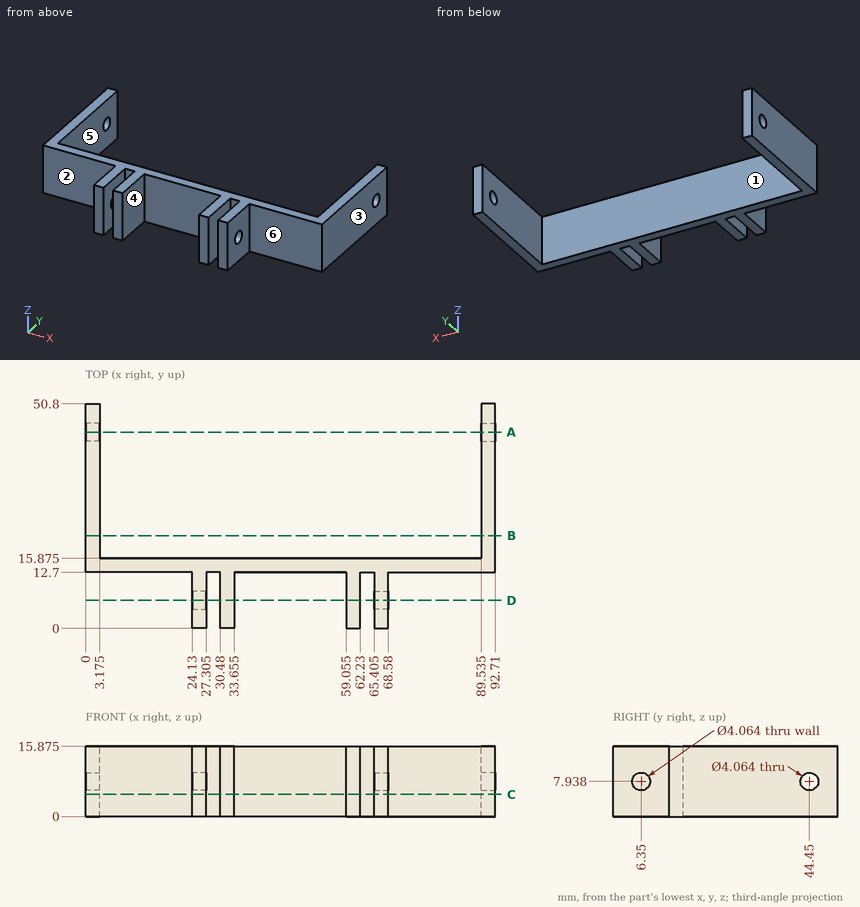
Part print with two shaded views. Sizes in mm from the minimum x, y, z corner. A direction names the side the tool comes from. Give positions to 0.01 mm unless a question says otherwise; leave off trailing zeros. Order: outer loops, then holes, each group sorted by start corner. A loop starts at its lowest first (then second) coordinate and runs counter-clockwise, first axis right, second up.
(1) Saw through at D-D, the plane y = 6.35. Give the cut face in (x, z) (1 decimal).
(2) Drill centre lines: L1, parallel to X at y = 12, z = 12.25 (1 decimal); L2, parallel to X at y = 16.5, z = 2.25 (1 decimal); L3, parallel to Z at x = 66.75, y = 6.35 (1 decimal). Where is each one in solid material? Low to high.
(3) Saw through at A-A, the plane y = 44.45. Give the cut face in (x, z) (1 decimal).
(4) Mould opens along X. For the marked faces 1, 2 and 3 say: released by +X, released by -X, zero draft, split by the parting line, or undercut.
(5) Saw through at C-C, the plane z = 5. Give the cut face in (x, y) (1 decimal).
(6) Tool access for the marked faces 4, 5 and 6: list every direction of +Z, -Z, +X, -X, +Y, -Y with a clear straight run to the whole face (end or side of a thin tool).
(7) Flat gauge pins, fed straight in: pin 1 (3.5 mm diameter, centred on y = 6.35, z = 7.94, fed in from +X); pin 2 (6.5 mm diameter, centred on y = 6.5, z = 5, fed in from +X); pin 3 (2.5 mm diameter, centred on y = 44.45, z = 7.94, fed in from +X); pin 4 (1 mm diameter, centred on x = 56.5, z = 8.5, fed in from +Y) (1 decimal). Where does each tip first touch, or does it go through?
(8) Saw through at B-B, the plane y = 21. Give the cut face in (x, z) (1 decimal), then the cut area to 3 significant figures.
Results found:
1. outline: (24.1, 0) - (27.3, 0) - (27.3, 5.9) - (24.1, 5.9) - close; (24.1, 10) - (27.3, 10) - (27.3, 15.9) - (24.1, 15.9) - close; (30.5, 0) - (33.7, 0) - (33.7, 15.9) - (30.5, 15.9) - close; (59.1, 0) - (62.2, 0) - (62.2, 15.9) - (59.1, 15.9) - close; (65.4, 0) - (68.6, 0) - (68.6, 5.9) - (65.4, 5.9) - close; (65.4, 10) - (68.6, 10) - (68.6, 15.9) - (65.4, 15.9) - close
2. L1: x = 24.1 to 27.3, 30.5 to 33.7, 59.1 to 62.2, 65.4 to 68.6
2. L2: x = 0 to 3.2, 89.5 to 92.7
2. L3: z = 0 to 5.9, 10 to 15.9
3. outline: (0, 0) - (3.2, 0) - (3.2, 5.9) - (0, 5.9) - close; (0, 10) - (3.2, 10) - (3.2, 15.9) - (0, 15.9) - close; (89.5, 0) - (92.7, 0) - (92.7, 5.9) - (89.5, 5.9) - close; (89.5, 10) - (92.7, 10) - (92.7, 15.9) - (89.5, 15.9) - close
4. face 1: undercut
4. face 2: zero draft
4. face 3: released by +X
5. outline: (0, 12.7) - (24.1, 12.7) - (24.1, 0) - (27.3, 0) - (27.3, 12.7) - (30.5, 12.7) - (30.5, 0) - (33.7, 0) - (33.7, 12.7) - (59.1, 12.7) - (59.1, 0) - (62.2, 0) - (62.2, 12.7) - (65.4, 12.7) - (65.4, 0) - (68.6, 0) - (68.6, 12.7) - (92.7, 12.7) - (92.7, 50.8) - (89.5, 50.8) - (89.5, 15.9) - (3.2, 15.9) - (3.2, 50.8) - (0, 50.8) - close
6. face 4: +Z, -Z, -Y
6. face 5: +Z, -Z, +Y
6. face 6: +Z, -Z, +X, -Y
7. pin 1: stops at x = 62.23
7. pin 2: stops at x = 68.58
7. pin 3: passes through
7. pin 4: stops at y = 15.9
8. outline: (0, 0) - (3.2, 0) - (3.2, 15.9) - (0, 15.9) - close; (89.5, 0) - (92.7, 0) - (92.7, 15.9) - (89.5, 15.9) - close
8. area: 101 mm2
